Autodesk Inventor part; units mm, degrees
ref_plane "Work Plane1" through (6.25, 0, 2) normal (0, 0, 1) x (1, 0, 0)
ref_plane "YZ Plane" through (0, 0, 0) normal (1, 0, 0) x (0, 1, 0)
ref_plane "XZ Plane" through (0, 0, 0) normal (0, 1, 0) x (-1, 0, 0)
sketch "Sketch1" plane through (0, 0, 0) normal (0, 0, 1) x (1, 0, 0)
  line L0 (-1.8, 0) -> (-1.8, 3.5)
  line L1 (-1.8, 3.5) -> (0, 3.5)
  line L2 (0, 3.5) -> (0, 2)
  line L3 (0, 2) -> (12.5, 2)
  line L4 (12.5, 2) -> (12.5, 0)
  line L5 (-1.8, 0) -> (12.5, 0)
  line L6 (-4.7305, 0) -> (15.7829, 0)
  line L7 (0, -1.84) -> (0, 4.39)
  circle A0 centre (10.25, 0) radius 0.95
  dimension "d0" = 4
  dimension "d1" = 7
  dimension "d2" = 1.8
  dimension "d3" = 12.5
  dimension "d5" = 2.25
  dimension "d6" = 1.9
revolve "Body" add sketch "Sketch1" angle 360 about axis through (-1.8, 0, 0) along (1, 0, 0) picked at (10.3623, 0.2961) contours L0 L1 L2 L7 L5 | L7 L3 L4 L5 A0 | A0 L5
extrude "Hole" [suppressed]
chamfer "Chamfer1" distance 0.5 angle 45 1 edges at (-1.8, -3.5, 0) measured on face at (-1.2, 3.4547, -0.5614)
chamfer "Chamfer2" distance 0.9 angle 20 1 edges at (12.5, -2, 0) measured on face at (4.1667, 1.9935, -0.1609)
ref_plane "Work Plane1" through (6.25, 0, 2) normal (0, 0, 1) x (1, 0, 0)
equation "\"d0\" = NND"
equation "\"d1\" = KOD"
equation "\"d2\" = KOH"
equation "\"d3\" = NLG"
equation "\"d5\" = DIST"
equation "\"d6\" = BOR"
equation "\"d7\" = NND"
equation "\"d9\" = PHH2"
equation "\"d10\" = FAWI2"
equation "\"d16\" = PHH2"
equation "\"d11\" = PHH1"
equation "\"d12\" = FAWI1"
equation "\"d17\" = PHH1"
equation "\"PHH1\" = 0.9"
equation "\"PHH2\" = 0.5"
equation "\"KOD\" = 7"
equation "\"KOH\" = 1.8"
equation "\"NND\" = 4"
equation "\"FAWI1\" = 20deg"
equation "\"FAWI2\" = 45deg"
equation "\"DIST\" = 2.25"
equation "\"BOR\" = 1.9"
equation "\"NLG\" = 12.5"
properties part number "DS51F1496-07" material "Steel, Mild"
The model under review builds one solid part; all positions refer to its coordinate system, in mm. A direction names the side the tool comes from. Give positions to 0.01 mm unless a question says otherwise; leave off trailing zeros. Order: outer loops, then holes, each group sorted by start corner. A loop starts at its lowest first (then second) coordinate and runs counter-clockwise, first axis right, second up. Notation, with made-up numbers: M 88.5,6 L 126.5,6 A26 cw 126.5,32 Z; hole C 48.5,84 d3. An arc over 180 degrees is marked long. Answer in a Markdown table with one row per item. Add a question column.
1. Machinability: for faces 1 (the cylindrical face through (6, 0, -2)), 2 (the flat face through (12.5, 0, 0)), which of the approach directions +Z, -Z, +X, -X, +Y, -Y give a long, thin tool a straight path to every point of the face, cutting with its end or side? Answer none if there is none.
2. To check wall thickness, follow line 1 along X through (y, z) = (1.5, 2.25); line 2 along Y through (x, z) = (0.5, -1); line 3 along X through (y, z) = (3, -1.25). State the ranges of each line that lie inside material, in increasing order.
3. Add section C-C on x = 1.5. State the section outline as (y, z) points.
4. Add section A-A on y = 0. State the section outline as (x, z) points, plus the area to 3 significant figures.
5. For pin 1 Ø2 at (x, z) = (5.5, 2) entering from +Y; pin 2 Ø2 at (x, y) = (1.5, 2) entering from +Z; pin 3 Ø3 at (x, z) = (9.5, 1.5) entering from +Y, all flat-tipped, find the tip position at first contact; note any pin that passes through.
The answers:
| question | item | result |
|---|---|---|
| 1 | face 1 | +X |
| 1 | face 2 | +Z, -Z, +X, +Y, -Y |
| 2 | line 1 | -1.8 to 0 |
| 2 | line 2 | -1.73 to 1.73 |
| 2 | line 3 | -1.55 to 0 |
| 3 | outline | C 0,0 d4 |
| 4 | outline | M -1.8,-3 L -1.3,-3.5 L 0,-3.5 L 0,-2 L 11.6,-2 L 12.5,-1.67 L 12.5,1.67 L 11.6,2 L 0,2 L 0,3.5 L -1.3,3.5 L -1.8,3 Z |
| 4 | area | 62.1 mm2 |
| 5 | pin 1 | y = 1.73 |
| 5 | pin 2 | z = 1.73 |
| 5 | pin 3 | y = 2 |
